Build history of the part. All positions in model axes, mm. A direction names the side the tool comes from. Round coordinates to 2 decimals unless told otherwise and drop trailing zeros. Write each loop counter-clockwise with the first axis right and the second up, starting at its lowest first coordinate (ties: lowest second). Pieces come first, ordered by that corner, then holes. Notation, with made-up numbers: M -6.75,3 L 4.25,3 A8 cw 4.25,11 Z; hole C 17.25,63 d1. An arc over 180 degrees is marked long. Write item = value, one per line.
from build123d import *

# Parameters (mm, degrees)
IZIM1_R                     = 9
IZIM1_R_2                   = 6.6
Y_KSEKLIK_EKSTR_ZYON1_DEPTH = 5
IZIM2_R                     = 9
IZIM2_R_2                   = 8
KES_EKSTR_ZYON1_DEPTH       = 3.9
IZIM3_R                     = 7.1
KES_EKSTR_ZYON2_DEPTH       = 1
L_O_ALTMA1_COUNT            = 2
L_O_ALTMA1_PITCH            = 4
RADYUS1_R                   = 0.2


with BuildPart() as part:
    # Çizim1 → Yükseklik-Ekstrüzyon1 (new body)
    with BuildSketch(Plane(origin=(0, 0, 0), x_dir=(1, 0, 0), z_dir=(0, 1, 0))):
        Circle(IZIM1_R)
        Circle(IZIM1_R_2, mode=Mode.SUBTRACT)
    extrude(amount=Y_KSEKLIK_EKSTR_ZYON1_DEPTH)

    # Çizim2 → Kes-Ekstrüzyon1 (cut)
    with BuildSketch(Plane(origin=(0, 5, 0), x_dir=(1, 0, 0), z_dir=(0, 1, 0))):
        Circle(IZIM2_R)
        Circle(IZIM2_R_2, mode=Mode.SUBTRACT)
    extrude(amount=-KES_EKSTR_ZYON1_DEPTH, mode=Mode.SUBTRACT)

    # Çizim3 → Kes-Ekstrüzyon2 (cut)
    with BuildSketch(Plane(origin=(0, 5, 0), x_dir=(1, 0, 0), z_dir=(0, 1, 0))):
        Circle(IZIM3_R)
    kes_ekstr_zyon2 = extrude(amount=-KES_EKSTR_ZYON2_DEPTH, mode=Mode.SUBTRACT)

    # LÇoğaltma1: Kes-Ekstrüzyon2 ×2
    with Locations(*[(0, -i * L_O_ALTMA1_PITCH, 0) for i in range(1, L_O_ALTMA1_COUNT)]):
        add(kes_ekstr_zyon2, mode=Mode.SUBTRACT)

    # Çizim5 → Kes-Döndür1 (revolve, cut)
    with BuildSketch(Plane.XY):
        Polygon((-6.975, 2.914213562), (-6.975, 2.085786438), (-5.889213562, 1), (-5.889213562, 4), align=None)
    revolve(axis=Axis((0, 0, 0), (0, 1, 0)), mode=Mode.SUBTRACT)

    # Radyus1
    radyus1_edges = [part.edges().sort_by_distance(p)[0] for p in [
        (-9, 1.1, 0),
        (-8, 5, 0),
        (-7.1, 5, 0),
        (-9, 0, 0),
        (-7.1, 0, 0),
    ]]
    fillet(radyus1_edges, radius=RADYUS1_R)


solid = part.part
1. Probe probe 1 along Z at (x, y) = (0, 3.55); probe 2 along Z at (x, y) = (0, 0.6); probe 3 along X at (y, z) = (4.35, 0). List the from-to ranges inside material, lowest first.
Responses:
probe_1 = -8 to -6.6, 6.6 to 8
probe_2 = -9 to -7.1, 7.1 to 9
probe_3 = -8 to -7.1, 7.1 to 8
2. Mould opens along Z. For faces 1 (the face through (-4.864, 1.35, -4.461)), 2 (the face through (-1.73, 2.98, 7.81)), 3 (the face through (3, 5, 7)), 4 (the face through (-0.92, 4.41, -7.04)) say: pulls with the +Z half, pulls with the -Z half, needs draft (parallel to the pull), parting line crosses it, or undercut.
Responses:
face_1 = undercut
face_2 = parting line crosses it
face_3 = needs draft
face_4 = undercut
3. Band-saw the part on A-A (y = 3.5). List the corners of the cut face in (x, z).
Responses:
outline = C 0,0 d16; hole C 0,0 d13.2
4. Tool access for faces 5 (the face through (1.51, 2.49, -6.81)), 6 (the face through (-0.92, 0.61, -7.04)), 7 (the face through (2, 1.1, 8)), 8 (the face through (-3, 0, -7)): list every direction of +Z, -Z, +X, -X, +Y, -Y with a clear straight run to the whole face (end or side of a thin tool).
Responses:
face_5 = none
face_6 = -Y
face_7 = +Y
face_8 = +Z, -Z, +X, -X, -Y
5. Flat gauge pin, fed straight in: pin 1 (3 mm diameter, centred on x = 5.5, y = 1, fed in from +Z). Where does the tip first touch, or does it go through?
Responses:
pin_1 = 8.06
